The listing builds one solid part. Answer for the finished solid, in the listing's coordinates (mm). A direction names the side the tool comes from. Coordinates: 2 decimals unless noted, no trailing zeros. Order: outer loops, then holes, each group sorted by start corner. A loop starts at its lowest first (then second) coordinate and runs counter-clockwise, first axis right, second up. Notation, with made-up numbers: (71, 0) -> (118, 0) arc R31 ccw to (118, 25) -> close; hole circle Ø9 at (53, -31.5). An arc over 180 degrees is marked (long way). Write each question's results on one line, items separated by ' | '. Start each with the question number.
(1) Given pin 1 (6 mm diameter, centred on x = -16, z = -10, fed in from +Y); pin 2 (6 mm diameter, centred on x = 3, y = 8.5, fed in from +Z); pin 3 (1 mm diameter, centred on y = 11.5, z = 3.5, fed in from +X); pin 4 (7.5 mm diameter, centred on x = 0, z = 0, fed in from +Y), each flat-ended and moving along its own axis, determine where each tip first touches the part or whether it passes through.
(2) Straight lines are drawn through the part: L1, parallel to Z at x = 0, y = 6.5; L2, parallel to Y at x = 19.5, z = -3. For each, find the intervals that lie inside material, in ascending order.
(3) The part is cut by section C-C, the plane y = 10. Give the vertices of the cut face in (x, z), then the cut area to 3 significant figures.
(4) Determine the mould class of faces 3 (the face through (-6, 5, -6)), 4 (the face through (-25.865, 2.465, 10.724)), 5 (the face through (2.86, 6.9, -5.5)) for opening direction X: +X half, -X half, draft (parallel to the pull), parting line (faces both ways), or undercut.
(5) The part is cut by section A-A, the plane x = 0. Give the vertices of the cut face in (y, z), then the cut area to 3 significant figures.
(6) The part is cut by section B-B, the plane z = 0. Give the vertices of the cut face in (x, y), then the cut area to 3 significant figures.
(7) The part is cut by section D-D, the plane z = -16.5. Give the vertices of the cut face in (x, y), then the cut area to 3 significant figures.
(8) A tool of negligible diameter and unlimited length cuts with its end or side. For faces 1 (the face through (-1.73, 9.44, -7.81)), 2 (the face through (4, 14, 5)), from which of +Z, -Z, +X, -X, +Y, -Y can it reach the whole face along a straight path? Write none if from no direction.
Autodesk Inventor part; units mm, degrees
ref_plane "YZ Plane" through (0, 0, 0) normal (1, 0, 0) x (0, 1, 0)
ref_plane "XZ Plane" through (0, 0, 0) normal (0, 1, 0) x (-1, 0, 0)
ref_plane "XY Plane" through (0, 0, 0) normal (0, 0, 1) x (1, 0, 0)
sketch "スケッチ1" plane through (0, 0, 0) normal (0, 1, 0) x (-1, 0, 0)
  circle A0 centre (0, 0) radius 29.5
  circle A1 centre (0, 0) radius 28
  dimension "d0" = 59
  dimension "d10" = 56
extrude "押し出し1" add sketch "スケッチ1" along normal blind 5 contours A1
sketch "スケッチ2" plane through (0, 5, 0) normal (0, 1, 0) x (1, 0, 0)
  circle A0 centre (0, 0) radius 6.2
  circle A1 centre (0, 0) radius 8
  dimension "d3" = 16
  dimension "d9" = 12.4
extrude "押し出し2" cut sketch "スケッチ2" against normal blind 5 contours A0
extrude "押し出し3" add sketch "スケッチ2" along normal blind 9
properties part number "maingear"
Established:
1) pin 1: stops at y = 5 | pin 2: stops at z = 8 | pin 3: stops at x = 7.42 | pin 4: passes through
2) L1: z = -8 to -6.2, 6.2 to 8 | L2: y = 0 to 5
3) outline: circle Ø16 at (0, 0); hole circle Ø12.4 at (0, 0) | area: 80.3 mm^2
4) face 3: draft | face 4: parting line | face 5: undercut
5) outline: (0, -28) -> (5, -28) -> (5, -8) -> (14, -8) -> (14, -6.2) -> (0, -6.2) -> close; (0, 6.2) -> (14, 6.2) -> (14, 8) -> (5, 8) -> (5, 28) -> (0, 28) -> close | area: 250 mm^2
6) outline: (-28, 0) -> (-6.2, 0) -> (-6.2, 14) -> (-8, 14) -> (-8, 5) -> (-28, 5) -> close; (6.2, 0) -> (28, 0) -> (28, 5) -> (8, 5) -> (8, 14) -> (6.2, 14) -> close | area: 250 mm^2
7) outline: (-22.62, 0) -> (22.62, 0) -> (22.62, 5) -> (-22.62, 5) -> close | area: 226 mm^2
8) face 1: +Y | face 2: +Z, -Z, +X, -X, +Y
